```python
from build123d import *

# Parameters (mm, degrees)
SKETCH1_W           = 85
SKETCH1_H           = 160
BOSS_EXTRUDE1_DEPTH = 10
SKETCH2_W           = 8
SKETCH2_H           = 40
BOSS_EXTRUDE2_DEPTH = 20
SKETCH4_W           = 8
SKETCH4_H           = 40
BOSS_EXTRUDE3_DEPTH = 20
SKETCH3_R           = 2.5
CUT_EXTRUDE1_DEPTH  = 34


with BuildPart() as part:
    # Sketch1 → Boss-Extrude1 (new body)
    with BuildSketch(Plane.XY):
        with Locations((27.5, 76)):
            Rectangle(SKETCH1_W, SKETCH1_H)
    extrude(amount=BOSS_EXTRUDE1_DEPTH)

    # Sketch2 → Boss-Extrude2 (add)
    with BuildSketch(Plane.XY.offset(10)):
        with Locations((-11, 34.15)):
            Rectangle(SKETCH2_W, SKETCH2_H)
    extrude(amount=BOSS_EXTRUDE2_DEPTH)

    # Sketch4 → Boss-Extrude3 (add)
    with BuildSketch(Plane.XY.offset(10)):
        with Locations((15, 34.15)):
            Rectangle(SKETCH4_W, SKETCH4_H)
    extrude(amount=BOSS_EXTRUDE3_DEPTH)

    # Sketch3 → Cut-Extrude1 (cut)
    with BuildSketch(Plane.ZY.offset(15)):
        with Locations((20, 34.15)):
            Circle(SKETCH3_R)
    extrude(amount=-CUT_EXTRUDE1_DEPTH, mode=Mode.SUBTRACT)


solid = part.part
```
The model under review builds one solid part; all positions refer to its coordinate system, in mm. A direction names the side the tool comes from. Round coordinates to 2 decimals unless told otherwise and drop trailing zeros. Order: outer loops, then holes, each group sorted by start corner. A loop starts at its lowest first (then second) coordinate and runs counter-clockwise, first axis right, second up.
Item 1: Draft analysis for pull direction X (two halves, no side actions). For faces 5 (the flat face through (11, 29, 20)), 6 (the flat face through (27, 156, 5)), 7 (the flat face through (-15, 57, 8)), state which applies: released by +X, released by -X, zero draft, split by the parting line, or undercut.
Working result:
face 5: undercut
face 6: zero draft
face 7: released by -X
Item 2: To check wall thickness, follow probe 1 along Y at (x, z) = (-10.5, 20); probe 2 along X at (y, z) = (51, 16.75); probe 3 along Z at (x, y) = (16, 34). State the ranges of each line that lie inside material, in increasing order.
Working result:
probe 1: y = 14.15 to 31.65, 36.65 to 54.15
probe 2: x = -15 to -7, 11 to 19
probe 3: z = 0 to 17.5, 22.5 to 30
Item 3: Add section D-D, the plane x = 13. State the section outline as (y, z) points.
Working result:
outline: (-4, 0) - (156, 0) - (156, 10) - (54.15, 10) - (54.15, 30) - (14.15, 30) - (14.15, 10) - (-4, 10) - close; hole circle Ø5 at (34.15, 20)
Item 4: For pin 1 (2.5 mm diameter, centred on x = -11.5, z = 23, fed in from -Y); pin 2 (2 mm diameter, centred on x = 45, y = 119, fed in from +Z); pin 3 (10 mm diameter, centred on y = 41, z = 21.5, fed in from +X), all flat-tipped, find the tip position at first contact; note any pin that passes through.
Working result:
pin 1: stops at y = 14.15
pin 2: stops at z = 10
pin 3: stops at x = 19
Item 5: Add section C-C, the plane z = 20. State the section outline as (x, y) points.
Working result:
outline: (-15, 14.15) - (-7, 14.15) - (-7, 31.65) - (-15, 31.65) - close; (-15, 36.65) - (-7, 36.65) - (-7, 54.15) - (-15, 54.15) - close; (11, 14.15) - (19, 14.15) - (19, 31.65) - (11, 31.65) - close; (11, 36.65) - (19, 36.65) - (19, 54.15) - (11, 54.15) - close
Item 6: Add section A-A, the plane z = 27.5. State the section outline as (x, y) points, and give its area (3 significant figures).
Working result:
outline: (-15, 14.15) - (-7, 14.15) - (-7, 54.15) - (-15, 54.15) - close; (11, 14.15) - (19, 14.15) - (19, 54.15) - (11, 54.15) - close
area: 640 mm2
Item 7: Add section B-B, the plane y = 34.15. State the section outline as (x, z) points, and give its area (3 significant figures).
Working result:
outline: (-15, 0) - (70, 0) - (70, 10) - (19, 10) - (19, 17.5) - (11, 17.5) - (11, 10) - (-7, 10) - (-7, 17.5) - (-15, 17.5) - close; (-15, 22.5) - (-7, 22.5) - (-7, 30) - (-15, 30) - close; (11, 22.5) - (19, 22.5) - (19, 30) - (11, 30) - close
area: 1,090 mm2
Item 8: Machinability: for faces 1 (the flat face through (19, 29, 20)), 2 (the flat face through (15, 54.15, 20)), 3 (the flat face through (15, 14.15, 20)), 4 (the flat face through (-7, 29, 20)), which of the approach directions +Z, -Z, +X, -X, +Y, -Y give a long, thin tool a straight path to every point of the face, cutting with its end or side? Answer none if there is none.
Working result:
face 1: +Z, +X, +Y, -Y
face 2: +Z, +X, -X, +Y
face 3: +Z, +X, -X, -Y
face 4: +Z, +Y, -Y
